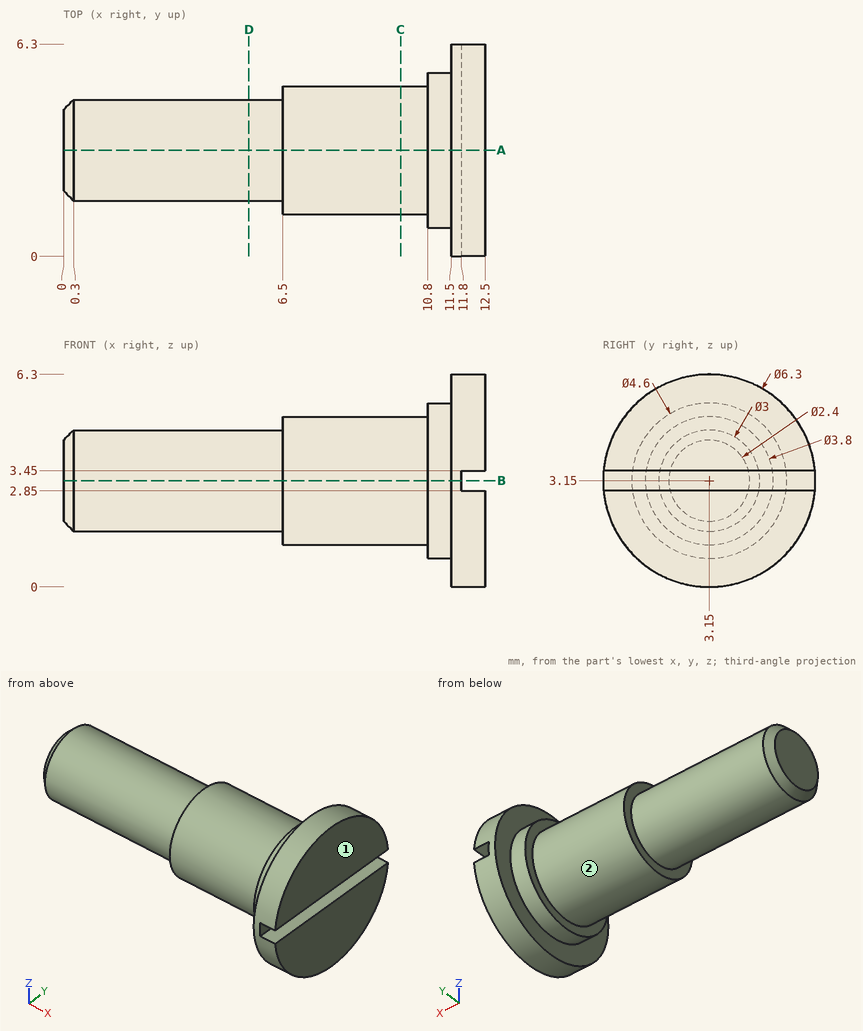
Here's the drawing with two shaded views (mm, measured from the low corner). I have some questions. A direction names the side the tool comes from. Give positions to 0.01 mm unless a question says otherwise; leave off trailing zeros. Write each loop counter-clockwise with the first axis right and the second up, starting at its lowest first coordinate (ties: lowest second). Pieces come first, ordered by that corner, then holes. Notation, with made-up numbers: (75, -30) -> (120, -30) arc R15 cw to (120, -16) -> close; hole circle Ø9 at (46, 57.5). An arc over 180 degrees is marked (long way). Answer as a JSON object with one key per item and string values. Group by question number.
Item 1: Suppose I cut it at C-C (x = 10). Please give me the cut outline in (y, z), plus the area to 3 significant figures.
Item 2: For the marked faces 1 and 2, which set-ups out of +Z, -Z, +X, -X, +Y, -Y let a thin tool reach every point of the face, with its end or its side?
Item 3: Suppose I cut it at B-B (z = 3.15). Please give me the cut outline in (x, y), plus the area to 3 significant figures.
Item 4: Please list where these lines run through material, in increasing order: line 1 (X direction, y = 1.5, z = 1.25); line 2 (X direction, y = 6, z = 3.25); line 3 (Z direction, x = 2.5, y = 3.25). Write a range as [from, to].
Item 5: I'm going to push flat-ended pins straight in: P1, Ø2, axis at x = 9.5, y = 1, coming from the +Z side; P2, Ø0.6, axis at x = 12, y = 2.5, coming from the -Z side; P3, Ø1.5, axis at x = 2, y = 3, coming from the +Z side. Where does each tip first touch, or does it pass through?
Item 6: Suppose I cut it at A-A (y = 3.15). Please give me the cut outline in (x, z).
Item 7: Suppose I cut it at D-D (x = 5.5). Please give me the cut outline in (y, z), plus the area to 3 significant figures.
Findings:
{
 "1": {"outline": "circle Ø3.8 at (3.15, 3.15)", "area": "11.3 mm²"},
 "2": {"face 1": "+Z, -Z, +X, +Y, -Y", "face 2": "-X"},
 "3": {"outline": "(0, 1.95) -> (0.3, 1.65) -> (6.5, 1.65) -> (6.5, 1.25) -> (10.8, 1.25) -> (10.8, 0.85) -> (11.5, 0.85) -> (11.5, 0) -> (11.8, 0) -> (11.8, 6.3) -> (11.5, 6.3) -> (11.5, 5.45) -> (10.8, 5.45) -> (10.8, 5.05) -> (6.5, 5.05) -> (6.5, 4.65) -> (0.3, 4.65) -> (0, 4.35) -> close", "area": "40.9 mm²"},
 "4": {"line 1": "x = [11.5, 12.5]", "line 2": "x = [11.5, 11.8]", "line 3": "z = [1.65, 4.65]"},
 "5": {"P1": "stops at z = 4.66", "P2": "stops at z = 0.02", "P3": "stops at z = 4.65"},
 "6": {"outline": "(0, 1.95) -> (0.3, 1.65) -> (6.5, 1.65) -> (6.5, 1.25) -> (10.8, 1.25) -> (10.8, 0.85) -> (11.5, 0.85) -> (11.5, 0) -> (12.5, 0) -> (12.5, 2.85) -> (11.8, 2.85) -> (11.8, 3.45) -> (12.5, 3.45) -> (12.5, 6.3) -> (11.5, 6.3) -> (11.5, 5.45) -> (10.8, 5.45) -> (10.8, 5.05) -> (6.5, 5.05) -> (6.5, 4.65) -> (0.3, 4.65) -> (0, 4.35) -> close"},
 "7": {"outline": "circle Ø3 at (3.15, 3.15)", "area": "7.07 mm²"}
}
